Read the model definition and answer for the solid it produces. Units are mm, in the model's axes. A direction names the side the tool comes from. Coordinates: 2 decimals unless noted, no trailing zeros. Loops run counter-clockwise (first coordinate to the right, second up) from the corner with the lowest first, then second, coordinate; pieces in that order, holes last. Notation, with made-up numbers: M -31,26 L 14,26 A34 ccw 14,56 Z; hole C -10.5,39.5 d11. An arc over 180 degrees is marked long. Put each result on its own line as item: value.
from build123d import *

# Parameters (mm, degrees)
BOSS_EXTRUDE1_DEPTH = 3
SKETCH2_R           = 2.25
CUT_EXTRUDE1_DEPTH  = 2
SKETCH4_W           = 11.97211786
SKETCH4_H           = 20
BOSS_EXTRUDE3_DEPTH = 4


with BuildPart() as part:
    # Sketch1 → Boss-Extrude1 (new, symmetric)
    with BuildSketch(Plane(origin=(0, 0, 0), x_dir=(1, 0, 0), z_dir=(0, 1, 0))):
        with BuildLine():
            Line((0, 61.2), (0, 51.2))
            ThreePointArc((0, 51.2), (20.599999205, 30.599999922), (-1.55e-07, 10))
            ThreePointArc((-1.55e-07, 10), (-5, 4.999999922), (0, 0))
            ThreePointArc((0, 0), (30.6, 30.6), (0, 61.2))
        make_face()
    extrude(amount=BOSS_EXTRUDE1_DEPTH, both=True)

    # Sketch2 → Cut-Extrude1 (cut)
    with BuildSketch(Plane(origin=(0, 3, 0), x_dir=(1, 0, 0), z_dir=(0, 1, 0))):
        with Locations(Location((0, 4.727516706, 0), (0, 0, 270))):
            Circle(SKETCH2_R)
    extrude(amount=-CUT_EXTRUDE1_DEPTH, mode=Mode.SUBTRACT)

    # Sketch4 → Boss-Extrude3 (add)
    with BuildSketch(Plane.ZY):
        with Locations((-56.2, 0)):
            Rectangle(SKETCH4_W, SKETCH4_H)
    extrude(amount=BOSS_EXTRUDE3_DEPTH)


solid = part.part
1) Find section D-D, the plane x = 3. Write down the section's boundary in (y, z).
Answer list:
outline: M -3,-61.05 L 3,-61.05 L 3,-50.98 L -3,-50.98 Z; M -3,-10.22 L 3,-10.22 L 3,-0.15 L -3,-0.15 Z
2) Given pin 1 Ø6 at (x, z) = (0, -4.73) entering from +Y; pin 2 Ø2 at (x, z) = (0.5, -4) entering from +Y; pin 3 Ø9.5 at (y, z) = (0, -53.5) entering from +X, each flat-ended and moving along its own axis, determine where each tip first touches the part or whether it passes through.
Answer list:
pin 1: stops at y = 3
pin 2: stops at y = 1
pin 3: stops at x = 24.64
3) Find section A-A, the plane y = -2. Write down the section's boundary in (x, z), plus the area to 3 significant figures.
Answer list:
outline: M -4,-62.19 L 0,-62.19 L 0,-61.2 A30.6 ccw 0,0 A5 ccw 0,-10 A20.6 cw 0,-51.2 L 0,-50.21 L -4,-50.21 Z
area: 891 mm^2
4) Determine the mould class of faces 1 (the cylindrical face through (20.595, 0.042, -31.053)), 2 (the flat face through (20, 3, -38)), 3 (the flat face through (0, 1, -5)), 4 (the flat face through (-2, 0, -62.186)) for opening direction Z: released by +Z, released by -Z, zero draft, split by the parting line, or undercut.
Answer list:
face 1: undercut
face 2: zero draft
face 3: undercut
face 4: released by -Z
5) Straight lines are drawn through the part: line 1 (Y direction, x = 21.5, z = -13.5); line 2 (Z direction, x = 2.5, y = -1); line 3 (Z direction, x = 7, y = 2). For each, find the intervals that lie inside material, in ascending order. Write a range as [from, to].
Answer list:
line 1: y = [-3, 3]
line 2: z = [-61.1, -51.05], [-10.15, -0.1]
line 3: z = [-60.39, -49.97], [-11.23, -0.81]
6) Which of the six approach directions +Z, -Z, +X, -X, +Y, -Y give full straight-line access (tool end or side, diameter ignored) to faces 5 (the flat face through (-4, 0, -56)), 6 (the cylindrical face through (30.593, 0.042, -29.927)), 7 (the cylindrical face through (0.676, 2.014, -2.581)), 8 (the flat face through (-2, 0, -50.214))?
Answer list:
face 5: -Z, -X, +Y, -Y
face 6: +X, +Y, -Y
face 7: +Y
face 8: -X, +Y, -Y
7) Find section C-C, the plane z = -5. Write down the section's boundary in (x, y), plus the area to 3 significant figures.
Answer list:
outline: M -5,-3 L 16.76,-3 L 16.76,3 L 2.23,3 L 2.23,1 L -2.23,1 L -2.23,3 L -5,3 Z
area: 122 mm^2
8) Find section B-B, the plane x = 10. Write down the section's boundary in (y, z), plus the area to 3 significant figures.
Answer list:
outline: M -3,-59.52 L 3,-59.52 L 3,-48.61 L -3,-48.61 Z; M -3,-12.59 L 3,-12.59 L 3,-1.68 L -3,-1.68 Z
area: 131 mm^2
